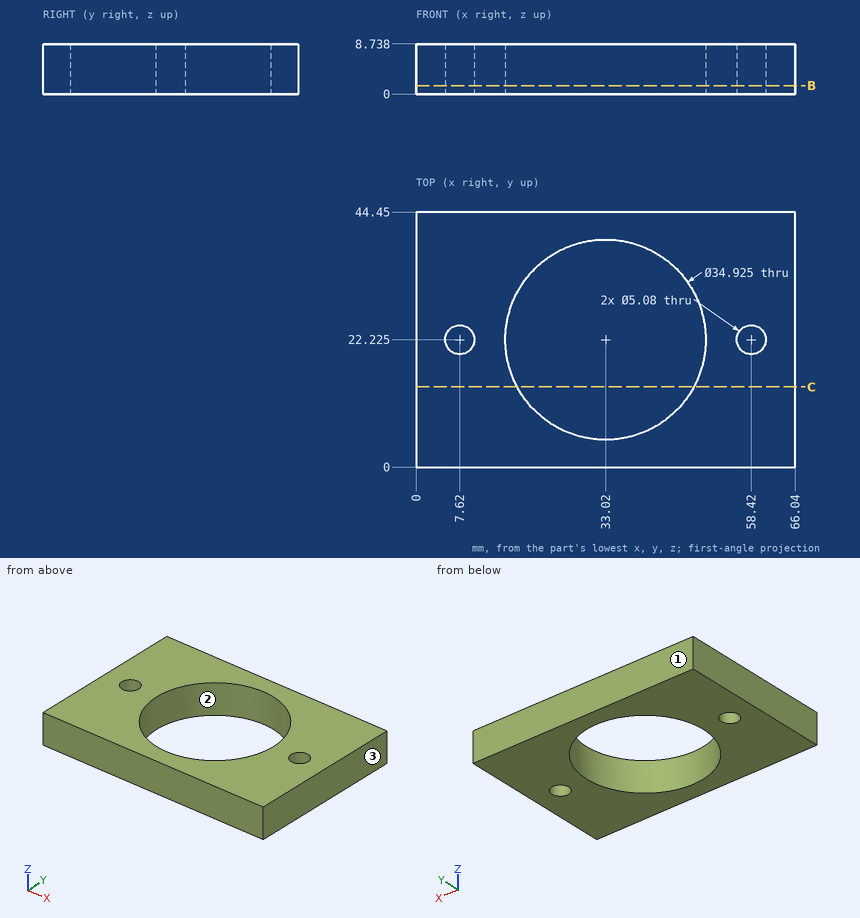
Check sheet for the drawn part. Datum: minimum x, y, z corner. Units: mm. Round coordinates to 2 decimals unless told otherwise and drop trailing zeros. Order: outer loops, then holes, each group sorted by start corner. A loop starts at its lowest first (then second) coordinate and runs counter-clockwise, first axis right, second up. Notation, with made-up numbers: (38.5, 30) - (65.5, 30) arc R33 ccw to (65.5, 62) - close; hole circle Ø1 at (64, 52.25). An arc over 180 degrees is marked (long way). Use a Markdown table: item, result. Add a question column.
(1) Sectioned sample at B-B, the plane z = 1.5. Count the separate pieces of the cut face and the enclosed holes in it, and give its area (3 significant figures).
(2) Release check for a two-part mould opening along Y. For the marked faces 1, 2 and 3 record: pulls with the +Y half, pulls with the -Y half, needs draft (parallel to the pull), parting line crosses it, or undercut.
(3) Material ranges on line 1 along Y through (x, z) = (33.5, 1.5); line 2 along X through (y, z) = (21.5, 1) (1 decimal); line 3 along X through (y, z) = (23, 2) (1 decimal), recorded low to high. Write a range as [from, to].
(4) Sectioned sample at C-C, the plane y = 14. Enter the section's corners in (x, z).
Answers below:
| question | item | result |
|---|---|---|
| 1 | separate pieces | 1 |
| 1 | enclosed holes | 3 |
| 1 | area | 1,940 mm² |
| 2 | face 1 | pulls with the +Y half |
| 2 | face 2 | undercut |
| 2 | face 3 | needs draft |
| 3 | line 1 | [0, 4.77], [39.68, 44.45] |
| 3 | line 2 | [0, 5.2], [10.1, 15.6], [50.5, 56], [60.9, 66] |
| 3 | line 3 | [0, 5.2], [10, 15.6], [50.5, 56], [60.8, 66] |
| 4 | outline | (0, 0) - (17.62, 0) - (17.62, 8.74) - (0, 8.74) - close; (48.42, 0) - (66.04, 0) - (66.04, 8.74) - (48.42, 8.74) - close |
